Read the model definition and answer for the solid it produces. Units are mm, in the model's axes. A direction names the side the tool comes from. Give positions to 0.01 mm unless a question says otherwise; leave off trailing zeros. Order: outer loops, then holes, each group sorted by start corner. A loop starts at its lowest first (then second) coordinate and runs counter-clockwise, first axis right, second up. Notation, with made-up numbers: (65.25, 65) - (78.25, 65) arc R14 cw to (78.25, 74) - close; hole circle Ø2 at (19.5, 44.5). An arc over 180 degrees is marked (long way). Write item = value, one per line.
Autodesk Inventor part; units mm, degrees
ref_plane "YZ Plane" through (0, 0, 0) normal (1, 0, 0) x (0, 1, 0)
ref_plane "XZ Plane" through (0, 0, 0) normal (0, 1, 0) x (-1, 0, 0)
ref_plane "XY Plane" through (0, 0, 0) normal (0, 0, 1) x (1, 0, 0)
sketch "Sketch1" plane through (0, 0, 0) normal (1, 0, 0) x (0, 1, 0)
  line L0 (0.0055, 3.1659) -> (2.7555, 1.5782)
  line L1 (2.7555, 1.5782) -> (2.7555, -1.5973)
  line L2 (2.7555, -1.5973) -> (0.0055, -3.185)
  line L3 (0.0055, -3.185) -> (-2.7445, -1.5973)
  line L4 (-2.7445, -1.5973) -> (-2.7445, 1.5782)
  line L5 (-2.7445, 1.5782) -> (0.0055, 3.1659)
  point P0 (0.0055, -0.0095)
  dimension "d1" = 5.5
extrude "Extrusion1" add sketch "Sketch1" along normal blind 31.56
sketch "Sketch2" plane through (0, 0, 0) normal (-1, 0, 0) x (0, 0, 1)
  circle A0 centre (0, 0) radius 1.5
  dimension "d4" = 3
extrude "Extrusion2" add sketch "Sketch2" along normal blind 6
sketch "Sketch3" plane through (31.56, 0, 0) normal (1, 0, 0) x (0, 0, -1)
  circle A0 centre (0, 0) radius 1.5
  dimension "d7" = 3
extrude "Extrusion3" cut sketch "Sketch3" against normal blind 6
properties part number "UpperSpacer"
1. For faces 5 (the face through (-2.96, -0.07, -1.5)), 6 (the face through (-6, 0, 0)), 7 (the face through (25.56, 0, 0)), determine the directions among +Z, -Z, +X, -X, +Y, -Y from which every point of the face is accessible in a straight line to the end or side of a thin tool.
Recorded:
face_5 = -X
face_6 = +Z, -Z, -X, +Y, -Y
face_7 = +X
2. Section B-B (x = 27) is taken. Determine the outline of the cut face in (y, z) (1 decimal).
Recorded:
outline = (-2.7, -1.6) - (0, -3.2) - (2.8, -1.6) - (2.8, 1.6) - (0, 3.2) - (-2.7, 1.6) - close; hole circle Ø3 at (0, 0)
3. Section A-A (z = 0) is taken. Determine the outline of the cut face in (x, y), and give its area (3 significant figures).
Recorded:
outline = (-6, -1.5) - (0, -1.5) - (0, -2.74) - (31.56, -2.74) - (31.56, -1.5) - (25.56, -1.5) - (25.56, 1.5) - (31.56, 1.5) - (31.56, 2.76) - (0, 2.76) - (0, 1.5) - (-6, 1.5) - close
area = 174 mm^2
4. Section C-C (x = 4.5) is taken. Determine the outline of the cut face in (y, z) (1 decimal), and give its area (3 significant figures).
Recorded:
outline = (-2.7, -1.6) - (0, -3.2) - (2.8, -1.6) - (2.8, 1.6) - (0, 3.2) - (-2.7, 1.6) - close
area = 26.2 mm^2
5. Determine the mould class of faces 1 (the face through (16, 2.756, 0)), 2 (the face through (0, -1.3, -1.4)), 3 (the face through (16, -2.744, 0)), 4 (the face through (28.6, 0.07, 1.5)) for opening direction Y: +Y half, -Y half, draft (parallel to the pull), parting line (faces both ways), or undercut.
Recorded:
face_1 = +Y half
face_2 = draft
face_3 = -Y half
face_4 = undercut
6. Straight lines are drawn through the part: L1, parallel to Y at x = 27, z = 0; L2, parallel to X at y = -1.05, z = 0; L3, parallel to X at y = -0.45, z = 1.5. For each, find the intervals that lie inside material, in ascending order. Write a range as [from, to].
Recorded:
L1 = [-2.74, -1.5], [1.5, 2.76]
L2 = [-6, 25.56]
L3 = [0, 31.56]
7. Flat-ended cylindrical pins translate along their axes: pin 1 (2.5 mm diameter, centred on y = 0, z = 0, fed in from +X); pin 2 (3 mm diameter, centred on y = 1.5, z = -1.5, fed in from -X); pin 3 (1 mm diameter, centred on x = 3.5, y = 1.5, fed in from -Z). Find the tip coordinate at first contact, or state that the pin passes through.
Recorded:
pin_1 = 25.56
pin_2 = -6
pin_3 = -2.61
8. Section D-D (y = 2.2) is taken. Determine the outline of the cut face in (x, z), and give its area (3 significant figures).
Recorded:
outline = (0, -1.92) - (31.56, -1.92) - (31.56, 1.9) - (0, 1.9) - close
area = 120 mm^2
